```python
from build123d import *

# Parameters (mm, degrees)
BOSS_EXTRUDE1_DEPTH      = 12
BOSS_EXTRUDE2_DEPTH      = 12
BOSS_EXTRUDE2_DEPTH_BACK = 8
SKETCH2_R                = 11.5
SKETCH2_R_2              = 4.625
SKETCH2_R_3              = 2.5
CUT_EXTRUDE1_DEPTH       = 62.308564335
CUT_EXTRUDE2_DEPTH       = 60.183951041
CUT_EXTRUDE2_DEPTH_BACK  = 4.45
SKETCH3_R                = 7.625
FILLET3_R                = 5
SKETCH4_R                = 4.75
CUT_EXTRUDE3_DEPTH       = 4


with BuildPart() as part:
    # Sketch1 → Boss-Extrude1 (new body)
    with BuildSketch(Plane(origin=(0, 0, 0), x_dir=(1, 0, 0), z_dir=(0, 1, 0))):
        Polygon((-22.5, 22.5), (-22.5, -22.5), (-24, -22.5), (-24, -37.605531925), (-11.25, -31.819805153), (-11.25, -22.5), (11.25, -22.5), (11.25, -31.819805153), (24, -37.605531925), (24, -22.5), (22.5, -22.5), (22.5, 22.5), (24, 22.5), (24, 37.605531925), (11.25, 31.819805153), (11.25, 22.5), (-11.25, 22.5), (-11.25, 31.819805153), (-24, 37.605531925), (-24, 22.5), align=None)
    extrude(amount=BOSS_EXTRUDE1_DEPTH)

    # Sketch1<3> → Boss-Extrude2 (add, two sides: drawn at the far end of the back side and taken through both)
    with BuildSketch(Plane(origin=(0, 0, 0), x_dir=(1, 0, 0), z_dir=(0, 1, 0)).offset(-BOSS_EXTRUDE2_DEPTH_BACK)):
        Polygon((-24, -37.605531925), (-24, -22.5), (-40.819805153, -22.5), (-40.819805153, -41.139805153), (-31.788474194, -41.139805153), align=None)
        Polygon((-40.819805153, 22.5), (-24, 22.5), (-24, 37.605531925), (-31.788474194, 41.139805153), (-40.819805153, 41.139805153), align=None)
        Polygon((24, -22.5), (24, -37.605531925), (31.788474194, -41.139805153), (40.819805153, -41.139805153), (40.819805153, -22.5), align=None)
        Polygon((31.788474194, 41.139805153), (24, 37.605531925), (24, 22.5), (40.819805153, 22.5), (40.819805153, 41.139805153), align=None)
    extrude(amount=BOSS_EXTRUDE2_DEPTH + BOSS_EXTRUDE2_DEPTH_BACK)

    # Sketch2 → Cut-Extrude1 (cut, through all)
    with BuildSketch(Plane(origin=(0, 12, 0), x_dir=(1, 0, 0), z_dir=(0, 1, 0))):
        with Locations(Location((0, 0, 0), (0, 0, 270))):
            Circle(SKETCH2_R)
        with Locations(Location((-31.819805153, 31.819805153, 0), (0, 0, 270))):
            Circle(SKETCH2_R_2)
        with Locations(Location((31.819805153, 31.819805153, 0), (0, 0, 270))):
            Circle(SKETCH2_R_2)
        with Locations(Location((31.819805153, -31.819805153, 0), (0, 0, 270))):
            Circle(SKETCH2_R_2)
        with Locations(Location((-31.819805153, -31.819805153, 0), (0, 0, 270))):
            Circle(SKETCH2_R_2)
        with Locations(Location((0, 17.5, 0), (0, 0, 270))):
            Circle(SKETCH2_R_3)
        with Locations(Location((17.5, 0, 0), (0, 0, 270))):
            Circle(SKETCH2_R_3)
        with Locations(Location((0, -17.5, 0), (0, 0, 270))):
            Circle(SKETCH2_R_3)
        with Locations(Location((-17.5, 0, 0), (0, 0, 270))):
            Circle(SKETCH2_R_3)
    extrude(amount=-CUT_EXTRUDE1_DEPTH, mode=Mode.SUBTRACT)

    # Sketch3 → Cut-Extrude2 (cut, two sides: drawn at the far end of the back side and taken through both)
    with BuildSketch(Plane.XZ.offset(-CUT_EXTRUDE2_DEPTH_BACK)):
        with Locations(Location((31.819805153, -31.819805153, 0), (0, 0, 270))):
            Circle(SKETCH3_R)
        with Locations(Location((-31.819805153, -31.819805153, 0), (0, 0, 270))):
            Circle(SKETCH3_R)
        with Locations(Location((-31.819805153, 31.819805153, 0), (0, 0, 270))):
            Circle(SKETCH3_R)
        with Locations(Location((31.819805153, 31.819805153, 0), (0, 0, 270))):
            Circle(SKETCH3_R)
    extrude(amount=CUT_EXTRUDE2_DEPTH + CUT_EXTRUDE2_DEPTH_BACK, mode=Mode.SUBTRACT)

    # Fillet3
    fillet3_edges = [part.edges().sort_by_distance(p)[0] for p in [
        (11.25, 6, 31.819805153),
        (11.25, 6, 22.5),
        (-11.25, 6, 22.5),
        (-11.25, 6, 31.819805153),
        (-11.25, 6, -31.819805153),
        (-11.25, 6, -22.5),
        (11.25, 6, -22.5),
        (11.25, 6, -31.819805153),
    ]]
    fillet(fillet3_edges, radius=FILLET3_R)

    # Sketch4 → Cut-Extrude3 (cut)
    with BuildSketch(Plane(origin=(0, 12, 0), x_dir=(1, 0, 0), z_dir=(0, 1, 0))):
        with Locations(Location((0, 17.5, 0), (0, 0, 270))):
            Circle(SKETCH4_R)
        with Locations(Location((17.5, 0, 0), (0, 0, 270))):
            Circle(SKETCH4_R)
        with Locations(Location((0, -17.5, 0), (0, 0, 270))):
            Circle(SKETCH4_R)
        with Locations(Location((-17.5, 0, 0), (0, 0, 270))):
            Circle(SKETCH4_R)
    extrude(amount=-CUT_EXTRUDE3_DEPTH, mode=Mode.SUBTRACT)


solid = part.part
```
Here's how the part is built. I have some questions about the finished solid (model axes, mm). A direction names the side the tool comes from. Give positions to 0.01 mm unless a question says otherwise; leave off trailing zeros. Order: outer loops, then holes, each group sorted by start corner. A loop starts at its lowest first (then second) coordinate and runs counter-clockwise, first axis right, second up. Notation, with made-up numbers: M -36.75,43.25 L -7.75,43.25 A18 ccw -7.75,49.25 Z; hole C 46,-34.75 d7. An arc over 180 degrees is marked long. Use a Markdown table: item, result. Add a question column.
1. Suppose I cut it at B-B (y = -2.5). List the corners of the cut face in (x, z) for me (3 decimals), and give its area (3 significant figures).
2. I need wall thicknesses on probe 1 along X at (y, z) = (2.5, -27.5); probe 2 along Z at (x, y) = (-3, 11); probe 3 along X at (y, z) = (2.25, -17.5). Which ranges of each line are inside material? Lowest first, please. Write a range as from..to.
3. Suppose I cut it at A-A (z = -17.5). List the corners of the cut face in (x, y) for me, and give its area (3 significant figures).
4. If we mould it in two halves opening along X, with no side actions, what happens to faces 1 (the flat face through (0, 6, 22.5)), 2 (the flat face through (22.5, 6, 0)), 3 (the flat face through (-40, -8, -32)), 4 (the cylindrical face through (20, 4, 0))? For each: +X half, -X half, draft (parallel to the pull), parting line (faces both ways), or undercut.
5. On a 3-axis mill with a long thin cutter (end or side, diameter ignored), from which of +Z, -Z, +X, -X, +Y, -Y can I reach the whole of each face in a straight line? I mean faces 5 (the flat face through (-24, -4, 30)), 6 (the flat face through (-32, 2, -22.5)), 7 (the cylindrical face through (9.75, 6.08, 23.93)). Say none if no direction works.
6. Suppose I cut it at C-C (x = 0). List the corners of the cut face in (y, z) for me.
7. Suppose I cut it at D-D (z = 0). List the corners of the cut face in (x, y) for me.
8. For pin 1 Ø3 at (x, z) = (0, 17.5) entering from +Y; pin 2 Ø10.5 at (x, z) = (-31.82, 31.82) entering from +Y; pin 3 Ø7.5 at (x, z) = (35.5, 31) entering from -Y; pin 4 Ø5.5 at (x, z) = (0, 17.5) entering from +Y, each with a flat end and sliding along its axis, tell me the tip position at first contact or that it passes through.
Results list:
| question | item | result |
|---|---|---|
| 1 | outline | M -40.82,-41.14 L -31.788,-41.14 L -24,-37.606 L -24,-22.5 L -40.82,-22.5 Z; M -40.82,22.5 L -24,22.5 L -24,37.606 L -31.788,41.14 L -40.82,41.14 Z; M 24,-37.606 L 31.788,-41.14 L 40.82,-41.14 L 40.82,-22.5 L 24,-22.5 Z; M 24,22.5 L 40.82,22.5 L 40.82,41.14 L 31.788,41.14 L 24,37.606 Z; hole C -31.82,-31.82 d15.25; hole C -31.82,31.82 d15.25; hole C 31.82,-31.82 d15.25; hole C 31.82,31.82 d15.25 |
| 1 | area | 468 mm² |
| 2 | probe 1 | x = -40.82..-38.1, -25.54..-11.25, 11.25..25.54, 38.1..40.82 |
| 2 | probe 2 | z = -22.5..-21.18, -13.82..-11.1, 11.1..13.82, 21.18..22.5 |
| 2 | probe 3 | x = -22.5..-2.5, 2.5..22.5 |
| 3 | outline | M -22.5,0 L -2.5,0 L -2.5,8 L -4.75,8 L -4.75,12 L -22.5,12 Z; M 2.5,0 L 22.5,0 L 22.5,12 L 4.75,12 L 4.75,8 L 2.5,8 Z |
| 3 | area | 462 mm² |
| 4 | face 1 | undercut |
| 4 | face 2 | +X half |
| 4 | face 3 | draft |
| 4 | face 4 | undercut |
| 5 | face 5 | +Z, -Z, -Y |
| 5 | face 6 | -X, +Y, -Y |
| 5 | face 7 | +Z, +Y, -Y |
| 6 | outline | M 0,-22.5 L 12,-22.5 L 12,-22.25 L 8,-22.25 L 8,-20 L 0,-20 Z; M 0,-15 L 8,-15 L 8,-12.75 L 12,-12.75 L 12,-11.5 L 0,-11.5 Z; M 0,11.5 L 12,11.5 L 12,12.75 L 8,12.75 L 8,15 L 0,15 Z; M 0,20 L 8,20 L 8,22.25 L 12,22.25 L 12,22.5 L 0,22.5 Z |
| 7 | outline | M -22.5,0 L -20,0 L -20,8 L -22.25,8 L -22.25,12 L -22.5,12 Z; M -15,0 L -11.5,0 L -11.5,12 L -12.75,12 L -12.75,8 L -15,8 Z; M 11.5,0 L 15,0 L 15,8 L 12.75,8 L 12.75,12 L 11.5,12 Z; M 20,0 L 22.5,0 L 22.5,12 L 22.25,12 L 22.25,8 L 20,8 Z |
| 8 | pin 1 | passes through |
| 8 | pin 2 | stops at y = 12 |
| 8 | pin 3 | stops at y = 4.45 |
| 8 | pin 4 | stops at y = 8 |
